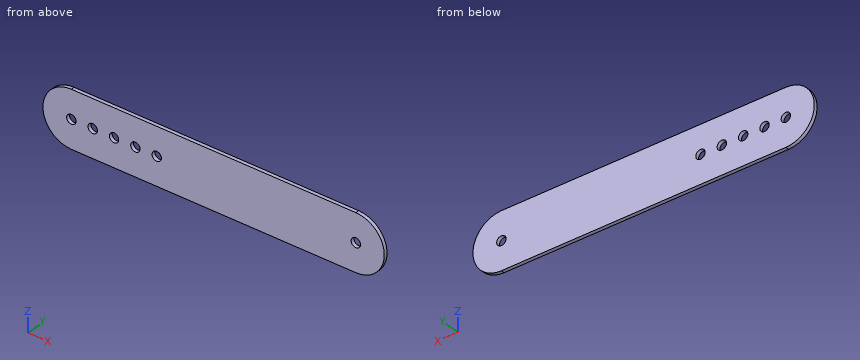
```python
from build123d import *

# Parameters (mm, degrees)
BOSS_EXTRUDE1_DEPTH = 3.175
SKETCH3_R           = 4.191
CUT_EXTRUDE1_DEPTH  = 281.570134948
LPATTERN1_OUTLINE_R = 4.191
LPATTERN1_DEPTH     = 3.175


# Read off the part's stored shape, not the designer's step: LPattern1
with BuildPart() as part:
    # Sketch1 → Boss-Extrude1 (new body)
    with BuildSketch(Plane(origin=(0, 0, 0), x_dir=(1, 0, 0), z_dir=(0, 1, 0))):
        with BuildLine():
            Line((0, 25.4), (-254, 25.4))
            ThreePointArc((-254, 25.4), (-279.4, 0), (-254, -25.4))
            Line((-254, -25.4), (0, -25.4))
            ThreePointArc((0, -25.4), (25.4, 0), (0, 25.4))
        make_face()
    extrude(amount=BOSS_EXTRUDE1_DEPTH)

    # Sketch3 → Cut-Extrude1 (cut, through all)
    with BuildSketch(Plane(origin=(0, 3.175, 0), x_dir=(1, 0, 0), z_dir=(0, 1, 0))):
        with Locations(Location((0, 0, 0), (0, 0, 270))):
            Circle(SKETCH3_R)
        with Locations(Location((-254, 0, 0), (0, 0, 270))):
            Circle(SKETCH3_R)
    extrude(amount=-CUT_EXTRUDE1_DEPTH, mode=Mode.SUBTRACT)

    # LPattern1 outline → LPattern1 (cut)
    with BuildSketch(Plane(origin=(0, 0, 0), x_dir=(1, 0, 0), z_dir=(0, 1, 0))):
        with Locations((-177.8, 0)):
            Circle(LPATTERN1_OUTLINE_R)
        with Locations((-196.85, 0)):
            Circle(LPATTERN1_OUTLINE_R)
        with Locations((-215.9, 0)):
            Circle(LPATTERN1_OUTLINE_R)
        with Locations((-234.95, 0)):
            Circle(LPATTERN1_OUTLINE_R)
    extrude(amount=LPATTERN1_DEPTH, mode=Mode.SUBTRACT)


solid = part.part
```
Verification items for the finished model (mm, model axes). Coordinates: 2 decimals unless noted, no trailing zeros. Write each loop counter-clockwise with the first axis right and the second up, starting at its lowest first coordinate (ties: lowest second). Pieces come first, ordered by that corner, then holes. Notation, with made-up numbers: M 20,-36 L 43,-36 A15 cw 43,-16 Z; hole C 64.25,55.5 d1. An arc over 180 degrees is marked long. One line per item, written item: value.
Item 1: Section check C-C, the plane y = 1.6. Record the boundary of the cut face in (x, z), plus the area to 3 significant figures.
Check sheet entries:
outline: M -254,-25.4 L 0,-25.4 A25.4 ccw 0,25.4 L -254,25.4 A25.4 ccw Z; hole C -254,0 d8.38; hole C -234.95,0 d8.38; hole C -215.9,0 d8.38; hole C -196.85,0 d8.38; hole C -177.8,0 d8.38; hole C 0,0 d8.38
area: 14,600 mm^2
Item 2: Section check A-A, the plane z = 0. Record the boundary of the cut face in (x, y) (3 decimals), plus the area to 3 significant figures.
Check sheet entries:
outline: M -279.4,0 L -258.191,0 L -258.191,3.175 L -279.4,3.175 Z; M -249.809,0 L -239.141,0 L -239.141,3.175 L -249.809,3.175 Z; M -230.759,0 L -220.091,0 L -220.091,3.175 L -230.759,3.175 Z; M -211.709,0 L -201.041,0 L -201.041,3.175 L -211.709,3.175 Z; M -192.659,0 L -181.991,0 L -181.991,3.175 L -192.659,3.175 Z; M -173.609,0 L -4.191,0 L -4.191,3.175 L -173.609,3.175 Z; M 4.191,0 L 25.4,0 L 25.4,3.175 L 4.191,3.175 Z
area: 808 mm^2
Item 3: Scan lines: line 1 along Z through (x, y) = (-215.9, 1.75); line 2 along Z through (x, y) = (-255, 1.15); line 3 along Z through (x, y) = (-265, 0.1). Record each from-to range of solid material in increasing order.
Check sheet entries:
line 1: z = -25.4 to -4.19, 4.19 to 25.4
line 2: z = -25.38 to -4.07, 4.07 to 25.38
line 3: z = -22.89 to 22.89
Item 4: Section check D-D, the plane z = 18.5. Record the boundary of the cut face in (x, y) (3 decimals).
Check sheet entries:
outline: M -271.404,0 L 17.404,0 L 17.404,3.175 L -271.404,3.175 Z
Item 5: Gauge pin test, flat ends, axial feed: pin 1 Ø1.5 at (y, z) = (1.5, -19.5) entering from +X; pin 2 Ø1.5 at (y, z) = (1, -5.5) entering from -X. Record the tip position at first contact, or that the pin passes through.
Check sheet entries:
pin 1: stops at x = 17.13
pin 2: stops at x = -278.95
Item 6: Section check B-B, the plane x = -196.85. Record the boundary of the cut face in (y, z) (3 decimals), plus the area to 3 significant figures.
Check sheet entries:
outline: M 0,-25.4 L 3.175,-25.4 L 3.175,-4.191 L 0,-4.191 Z; M 0,4.191 L 3.175,4.191 L 3.175,25.4 L 0,25.4 Z
area: 135 mm^2
